Design review of the part built by this model. Coordinates are the model's own, in mm. Face numbers are marked on the shaded views. A direction names the side the tool comes from. Coordinates: 2 decimals unless noted, no trailing zeros. Loops run counter-clockwise (first coordinate to the right, second up) from the corner with the lowest first, then second, coordinate; pieces in that order, holes last. Notation, with made-up numbers: M 4,89 L 63,89 A28 ccw 63,108 Z; hole C -28,38.5 d4. An arc over 180 degrees is marked long. One line per item, written item: value.
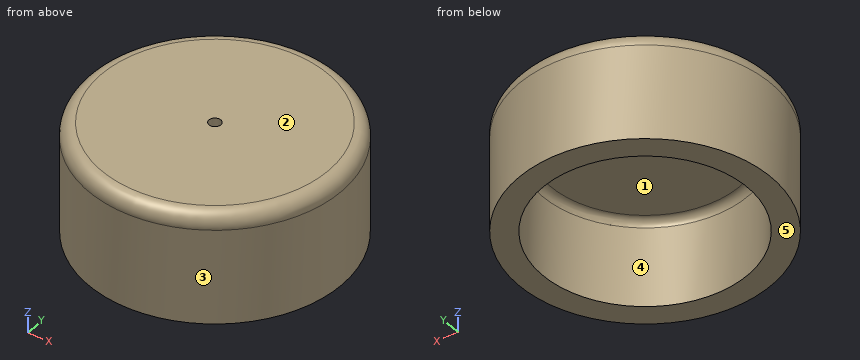
```python
from build123d import *

# Parameters (mm, degrees)
F2_R     = 3.175
F3_DEPTH = 25.4


with BuildPart() as f1:
    # F0 (on Front) → F1 (revolve)
    with BuildSketch(Plane.XZ):
        with BuildLine():
            Line((-71.568562, 56.310103), (-71.568562, 43.610103))
            Line((-71.568562, 43.610103), (-20.768562, 43.610103))
            ThreePointArc((-20.768562, 43.610103), (-17.985365, 42.542987), (-16.629005, 39.888706))
            Line((-16.629005, 39.888706), (-16.629005, -2.770737))
            Line((-16.629005, -2.770737), (-3.929005, -2.770737))
            Line((-3.929005, -2.770737), (-3.929005, 48.029263))
            ThreePointArc((-3.929005, 48.029263), (-5.481125, 53.790795), (-10.890138, 56.310103))
            Line((-10.890138, 56.310103), (-71.568562, 56.310103))
        make_face()
    revolve(axis=Axis((-71.568562, 0, 49.960103), (0, 0, 1)))

    # F2 (on face) → F3 (cut)
    with BuildSketch(Plane.XY.offset(56.310103)):
        with Locations((-71.568562, 0)):
            Circle(F2_R)
    extrude(amount=-F3_DEPTH, mode=Mode.SUBTRACT)


solid = f1.part
```
(1) Mouldability with a two-part tool opening along X and no side actions: class the marked faces 3, 4 and 5 as released by +X, released by -X, zero draft, split by the parting line, or undercut.
Reply:
face 3: split by the parting line
face 4: undercut
face 5: zero draft
(2) We need section A-A on y = 0. State the section outline as (x, z) points, then the cut area to 3 significant figures.
Reply:
outline: M -139.21,-2.77 L -126.51,-2.77 L -126.51,39.89 A4.16 cw -122.37,43.61 L -74.74,43.61 L -74.74,56.31 L -132.25,56.31 A7.07 ccw -139.21,48.03 Z; M -68.39,43.61 L -20.77,43.61 A4.16 cw -16.63,39.89 L -16.63,-2.77 L -3.93,-2.77 L -3.93,48.03 A7.07 ccw -10.89,56.31 L -68.39,56.31 Z
area: 2,800 mm2
(3) To check wall thickness, follow line 1 along Z through (x, y) = (-53, -38); line 2 along Y through (x, z) = (-79.5, 43); line 3 along X through (y, z) = (48, 24). State the ranges of each line that lie inside material, in increasing order. Write a range as [from, to].
Reply:
line 1: z = [43.61, 56.31]
line 2: y = [-67.17, -52.37], [52.37, 67.17]
line 3: x = [-119.22, -98.3], [-44.84, -23.91]
(4) Tool access review of the marked faces 1 and 2: name each direction out of +Z, -Z, +X, -X, +Y, -Y from which nothing blocks a thin tool from reaching the whole face with its end or side.
Reply:
face 1: -Z
face 2: +Z, +X, -X, +Y, -Y
(5) We need section B-B on z = 3. State the section outline as (x, y) points.
Reply:
outline: C -71.57,0 d135.28; hole C -71.57,0 d109.88
(6) Insertion check: pin 1 (3 mm diameter, centred on x = -81.5, z = 15.5, fed in from +Y); pin 2 (5 mm diameter, centred on y = -5.5, z = 24, fed in from -X); pin 3 (10 mm diameter, centred on y = -5, z = 19, fed in from -X). Each pin has a flat end and moves straight along its axis. Give the tip position at first contact, or say it passes through.
Reply:
pin 1: stops at y = 67.11
pin 2: stops at x = -139.14
pin 3: stops at x = -139.21
